CAD build for the part. Positions are in the model's coordinates, mm. Coordinates: 2 decimals unless noted, no trailing zeros. Loops run counter-clockwise (first coordinate to the right, second up) from the corner with the lowest first, then second, coordinate; pieces in that order, holes last. Notation, with made-up numbers: (-8.75, 22.25) -> (4.25, 22.25) arc R7 ccw to (4.25, 34.25) -> close; hole circle Ø9 at (20, 62). An arc over 180 degrees is marked (long way). Write each question's results on one line, items separated by ' | '.
```python
from build123d import *

# Parameters (mm, degrees)
CUT_EXTRUDE1_DEPTH       = 20
CUT_EXTRUDE1_DEPTH_BACK  = 20
SKETCH3_W                = 20
SKETCH3_H                = 10
SHELL1_T                 = -1
BOSS_EXTRUDE1_REACH      = 20.547
BOSS_EXTRUDE1_END_RADIUS = 10
SKETCH5_R                = 10


with BuildPart() as part:
    # Sketch2 → Revolve1 (revolve)
    with BuildSketch(Plane.XY):
        with BuildLine():
            Line((0, -10), (0, 10))
            ThreePointArc((0, 10), (10, 0), (0, -10))
        make_face()
    revolve(axis=Axis((0, -10, 0), (0, 1, 0)))

    # Sketch3 → Cut-Extrude1 (cut, two sides: drawn at the far end of the back side and taken through both)
    with BuildSketch(Plane(origin=(0, 0, 0), x_dir=(0, 0, -1), z_dir=(1, 0, 0)).offset(-CUT_EXTRUDE1_DEPTH_BACK)):
        with Locations((0, 7)):
            Rectangle(SKETCH3_W, SKETCH3_H)
    extrude(amount=CUT_EXTRUDE1_DEPTH + CUT_EXTRUDE1_DEPTH_BACK, mode=Mode.SUBTRACT)

    # Shell1
    shell1_openings = [part.faces().sort_by_distance(p)[0] for p in [
        (0, 2, 0),
    ]]
    offset(amount=SHELL1_T, openings=shell1_openings, kind=Kind.INTERSECTION)

    # Boss-Extrude1: up to this sphere (the profile starts outside it)
    boss_extrude1_end = Location((0, 0, 0)) * Sphere(BOSS_EXTRUDE1_END_RADIUS, mode=Mode.PRIVATE)
    # Sketch5 → Boss-Extrude1 (add, up to the surface)
    with BuildSketch(Plane(origin=(0, -10, 0), x_dir=(1, 0, 0), z_dir=(0, 1, 0)), mode=Mode.PRIVATE) as boss_extrude1_sk1:
        with Locations(Location((0, 0, 0), (0, 0, 90))):
            Circle(SKETCH5_R)
    boss_extrude1_tool1 = extrude(boss_extrude1_sk1.sketch, amount=BOSS_EXTRUDE1_REACH, mode=Mode.PRIVATE) - boss_extrude1_end
    add(boss_extrude1_tool1.solids().sort_by_distance((0, -10, 0))[0])


solid = part.part
```
Q1. Wall check: L1, parallel to X at y = -1, z = -2.5; L2, parallel to Z at x = -7, y = -4; L3, parallel to Z at x = 4.5, y = 1. Give the ranges that are in metal, low to high. Write a range as from..to.
Results are:
L1: -9.68..-8.59, 8.59..9.68 | L2: -7.14..-4, 4..7.14 | L3: -8.87..-7.73, 7.73..8.87
Q2. Cut at D-D on y = -7.75. Write the cut outline in (x, z).
Results are:
outline: circle Ø20 at (0, 0); hole circle Ø9.15 at (0, 0)
Q3. Cut at A-A on z = 0. Write the cut outline in (x, y).
Results are:
outline: (-10, -10) -> (10, -10) -> (10, 0) arc R10 ccw to (9.8, 2) -> (8.77, 2) arc R9 cw (long way) to (-8.77, 2) -> (-9.8, 2) arc R10 ccw to (-10, 0) -> close
Q4. Cut at C-C on y = -5. Write the cut outline in (x, z).
Results are:
outline: circle Ø20 at (0, 0); hole circle Ø14.97 at (0, 0)
Q5. Cut at B-B on x = -1.5. Write the cut outline in (y, z), and give its area (3 significant figures).
Results are:
outline: (-10, -9.89) -> (0, -9.89) arc R9.89 ccw to (2, -9.68) -> (2, -8.65) arc R8.87 cw (long way) to (2, 8.65) -> (2, 9.68) arc R9.89 ccw to (0, 9.89) -> (-10, 9.89) -> close | area: 78.1 mm^2
Q6. Drop flat-ended pins along their axis: pin 1 (2 mm diameter, centred on x = -6, y = -6.5, fed in from +Z); pin 2 (3 mm diameter, centred on y = -1, z = 3.5, fed in from +X); pin 3 (5 mm diameter, centred on y = -5, z = 5.5, fed in from -X). Give the stop position or say it passes through.
Results are:
pin 1: z = 8.66 | pin 2: x = 9.8 | pin 3: x = -9.54
